from build123d import *

# Parameters (mm, degrees)
BOSS_EXTRUDE2_DEPTH  = 1
SKETCH2_W            = 5
SKETCH2_H            = 47
BOSS_EXTRUDE3_DEPTH  = 2
FILLET2_R            = 5
FILLET2_OF_MIRROR2_R = 5
SKETCH3_R            = 1.5
BOSS_EXTRUDE5_DEPTH  = 100
SKETCH5_W            = 10
SKETCH5_H            = 8
BOSS_EXTRUDE6_DEPTH  = 1
FILLET3_R            = 3
SKETCH6_R            = 1
CUT_EXTRUDE1_DEPTH   = 1
FILLET3_OF_MIRROR4_R = 3


with BuildPart() as part:
    # Sketch1 → Boss-Extrude2 (new body)
    with BuildSketch(Plane.XY):
        Polygon((-45, 0), (45, 0), (40, 40), (-40, 40), align=None)
    extrude(amount=BOSS_EXTRUDE2_DEPTH)

    # Sketch2 → Boss-Extrude3 (add)
    with BuildSketch(Plane(origin=(21, 0, 0), x_dir=(0, 0, -1), z_dir=(1, 0, 0))):
        with Locations((-3.5, 23.5)):
            Rectangle(SKETCH2_W, SKETCH2_H)
    boss_extrude3 = extrude(amount=BOSS_EXTRUDE3_DEPTH)

    # Fillet2
    fillet2_edges = [part.edges().sort_by_distance(p)[0] for p in [
        (22, 0, 6),
    ]]
    fillet(fillet2_edges, radius=FILLET2_R)

    # Mirror2: Boss-Extrude3 across plane
    add(boss_extrude3.mirror(Plane(origin=(0, 0, 0), x_dir=(0, 0, 1), z_dir=(1, 0, 0))))

    # Fillet2 of Mirror2
    fillet2_of_mirror2_edges = [part.edges().sort_by_distance(p)[0] for p in [
        (-22, 0, 6),
    ]]
    fillet(fillet2_of_mirror2_edges, radius=FILLET2_OF_MIRROR2_R)

    # Sketch3 → Boss-Extrude5 (add)
    with BuildSketch(Plane(origin=(50, 0, 0), x_dir=(0, 0, -1), z_dir=(1, 0, 0))):
        with Locations((-3.5, 46)):
            Circle(SKETCH3_R)
    extrude(amount=-BOSS_EXTRUDE5_DEPTH)

    # Sketch5 → Boss-Extrude6 (add)
    with BuildSketch(Plane(origin=(0, 0, 0), x_dir=(1, 0, 0), z_dir=(0, 1, 0))):
        with Locations((-40, 4)):
            Rectangle(SKETCH5_W, SKETCH5_H)
    boss_extrude6 = extrude(amount=BOSS_EXTRUDE6_DEPTH)

    # Fillet3
    fillet3_edges = [part.edges().sort_by_distance(p)[0] for p in [
        (-35, 0.5, -8),
        (-45, 0.5, -8),
    ]]
    fillet(fillet3_edges, radius=FILLET3_R)

    # Sketch6 → Cut-Extrude1 (cut)
    with BuildSketch(Plane(origin=(0, 1, 0), x_dir=(1, 0, 0), z_dir=(0, 1, 0))):
        with Locations(Location((-40.376839828, 3.560660172, 0), (0, 0, 270))):
            Circle(SKETCH6_R)
    cut_extrude1 = extrude(amount=-CUT_EXTRUDE1_DEPTH, mode=Mode.SUBTRACT)

    # Mirror4: Boss-Extrude6, Cut-Extrude1 across plane
    add(boss_extrude6.mirror(Plane(origin=(0, 0, 0), x_dir=(0, 0, 1), z_dir=(1, 0, 0))))
    add(cut_extrude1.mirror(Plane(origin=(0, 0, 0), x_dir=(0, 0, 1), z_dir=(1, 0, 0))), mode=Mode.SUBTRACT)

    # Fillet3 of Mirror4
    fillet3_of_mirror4_edges = [part.edges().sort_by_distance(p)[0] for p in [
        (35, 0.5, -8),
        (45, 0.5, -8),
    ]]
    fillet(fillet3_of_mirror4_edges, radius=FILLET3_OF_MIRROR4_R)


solid = part.part
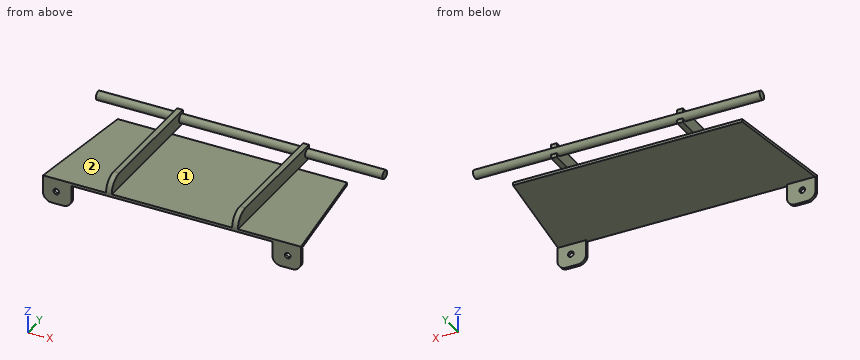
Could you check a few things on this model? Use its own coordinates, in mm. Face numbers are marked on the shaded views. Give positions to 0.01 mm unless a question says otherwise; leave off trailing zeros. Order: outer loops, then holes, each group sorted by start corner. A loop starts at its lowest first (then second) coordinate and runs counter-clockwise, first axis right, second up.
1. I need wall thicknesses on L1, parallel to X at y = 6, z = 4; L2, parallel to Z at x = 24.5, y = 27; L3, parallel to Y at x = -19.5, z = 3.5. Which ranges of each line are inside material? Lowest first, please.
2. Suppose I cut it at C-C (z = -6). List the corners of the cut face in (x, y) for me, plus the area to 3 significant figures.
3. We'd pull the mould along X, two halves only. Please class the marked faces 1 and 2: pulls with the +X half, pulls with the -X half, needs draft (parallel to the pull), parting line crosses it, or undercut.
4. Suppose I cut it at D-D (y = 22). List the corners of the cut face in (x, z) for me, plus the area to 4 significant figures.
5. Suppose I cut it at B-B (y = 46). List the corners of the cut face in (x, z) for me.
6. Will these pins go through, and if not, where does the flat tip stop? P1, Ø3, axis at x = 40.38, z = -3.56, coming from the +Y side; P2, Ø0.7, axis at x = 21.5, z = 5, coming from the +Y side; P3, Ø1.1, axis at x = -16.5, z = 0.5, coming from the +Y side.
7. Suppose I cut it at A-A (x = -11.5). List the corners of the cut face in (y, z) for me.
Solved:
1. L1: x = -23 to -21, 21 to 23
1. L2: z = 0 to 1
1. L3: y = 44.5 to 47.5
2. outline: (-44.83, 0) - (-35.17, 0) - (-35.17, 1) - (-44.83, 1) - close; (35.17, 0) - (44.83, 0) - (44.83, 1) - (35.17, 1) - close
2. area: 19.3 mm2
3. face 1: undercut
3. face 2: needs draft
4. outline: (-42.25, 0) - (42.25, 0) - (42.25, 1) - (23, 1) - (23, 6) - (21, 6) - (21, 1) - (-21, 1) - (-21, 6) - (-23, 6) - (-23, 1) - (-42.25, 1) - close
4. area: 104.5 mm2
5. outline: (-50, 2) - (-23, 2) - (-23, 1) - (-21, 1) - (-21, 2) - (21, 2) - (21, 1) - (23, 1) - (23, 2) - (50, 2) - (50, 5) - (23, 5) - (23, 6) - (21, 6) - (21, 5) - (-21, 5) - (-21, 6) - (-23, 6) - (-23, 5) - (-50, 5) - close
6. P1: stops at y = 1
6. P2: stops at y = 47
6. P3: stops at y = 40
7. outline: (0, 0) - (40, 0) - (40, 1) - (0, 1) - close; circle Ø3 at (46, 3.5)
